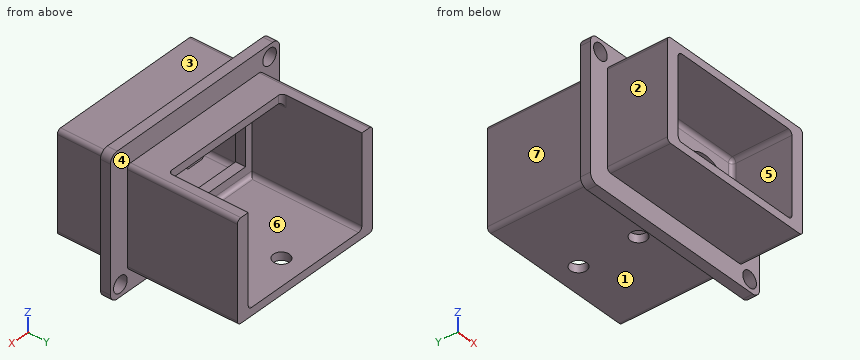
from build123d import *

# Parameters (mm, degrees)
SKETCH1_W                = 63.5
SKETCH1_H                = 44.45
BOSS_EXTRUDE1_DEPTH      = 3.175
FILLET3_R                = 2.54
BOSS_EXTRUDE3_DEPTH      = 19.05
BOSS_EXTRUDE3_DEPTH_BACK = 38.1
SKETCH3_W                = 50.8
SKETCH3_H                = 31.75
SKETCH3_W_2              = 42.672
SKETCH3_H_2              = 26.67
FILLET4_R                = 1.27
SKETCH4_W                = 42.672
SKETCH4_H                = 2.54
CUT_EXTRUDE1_DEPTH       = 25.4
FILLET5_R                = 1.27
FILLET6_R                = 1.27
CUT_EXTRUDE2_REACH       = 64.54
SKETCH5_R                = 2.5527
CUT_EXTRUDE3_REACH       = 56.347
SKETCH6_R                = 2.5527
FILLET7_R                = 1.27


with BuildPart() as part:
    # Sketch1 → Boss-Extrude1 (new body)
    with BuildSketch(Plane(origin=(0, 0, 0), x_dir=(1, 0, 0), z_dir=(0, 1, 0))):
        Rectangle(SKETCH1_W, SKETCH1_H)
        with BuildLine():
            Line((-19.05, -4.014611111), (-19.05, 9.525))
            Line((-19.05, 9.525), (19.05, 9.525))
            Line((19.05, 9.525), (19.05, -4.014611111))
            ThreePointArc((19.05, -4.014611111), (10.305774977, -9.455933485), (3.302, -1.905))
            Line((3.302, -1.905), (-3.302, -1.905))
            ThreePointArc((-3.302, -1.905), (-10.305774977, -9.455933485), (-19.05, -4.014611111))
        make_face(mode=Mode.SUBTRACT)
    extrude(amount=BOSS_EXTRUDE1_DEPTH)

    # Fillet3
    fillet3_edges = [part.edges().sort_by_distance(p)[0] for p in [
        (-31.75, 1.5875, 22.225),
        (-31.75, 1.5875, -22.225),
        (31.75, 1.5875, -22.225),
        (31.75, 1.5875, 22.225),
    ]]
    fillet(fillet3_edges, radius=FILLET3_R)

    # Sketch3 → Boss-Extrude3 (add, two sides: drawn at the far end of the back side and taken through both)
    with BuildSketch(Plane.XZ.offset(-BOSS_EXTRUDE3_DEPTH_BACK)):
        Rectangle(SKETCH3_W, SKETCH3_H)
        Rectangle(SKETCH3_W_2, SKETCH3_H_2, mode=Mode.SUBTRACT)
    extrude(amount=BOSS_EXTRUDE3_DEPTH + BOSS_EXTRUDE3_DEPTH_BACK)

    # Fillet4
    fillet4_edges = [part.edges().sort_by_distance(p)[0] for p in [
        (0, 0, -13.335),
        (21.336, 0, 0),
        (0, 0, 13.335),
        (-21.336, 0, 0),
        (-25.4, -9.525, -15.875),
        (-25.4, -9.525, 15.875),
        (25.4, -9.525, 15.875),
        (25.4, -9.525, -15.875),
        (-21.336, -9.525, 13.335),
        (21.336, -9.525, 13.335),
        (21.336, -9.525, -13.335),
        (-21.336, -9.525, -13.335),
    ]]
    fillet(fillet4_edges, radius=FILLET4_R)

    # Sketch4 → Cut-Extrude1 (cut)
    with BuildSketch(Plane(origin=(0, 38.1, 0), x_dir=(1, 0, 0), z_dir=(0, 1, 0))):
        with Locations((0, -14.605)):
            Rectangle(SKETCH4_W, SKETCH4_H)
    extrude(amount=-CUT_EXTRUDE1_DEPTH, mode=Mode.SUBTRACT)

    # Fillet5
    fillet5_edges = [part.edges().sort_by_distance(p)[0] for p in [
        (21.336, 12.7, 14.605),
        (-21.336, 12.7, 14.605),
        (-3.302, 1.5875, 1.905),
        (3.302, 1.5875, 1.905),
        (0, 3.175, -13.335),
        (21.336, 20.6375, -13.335),
        (-21.336, 20.6375, -13.335),
    ]]
    fillet(fillet5_edges, radius=FILLET5_R)

    # Fillet6
    fillet6_edges = [part.edges().sort_by_distance(p)[0] for p in [
        (0, 3.175, 13.335),
        (-21.336, 8.5725, 13.335),
        (21.336, 8.5725, 13.335),
    ]]
    fillet(fillet6_edges, radius=FILLET6_R)

    # Sketch5 → Cut-Extrude2 (cut, up to next)
    with BuildSketch(Plane(origin=(0, 0, -15.875), x_dir=(-1, 0, 0), z_dir=(0, 0, -1)), mode=Mode.PRIVATE) as cut_extrude2_sk1:
        with Locations((0, 11.557)):
            Circle(SKETCH5_R)
    cut_extrude2_tool1 = extrude(cut_extrude2_sk1.sketch, amount=-CUT_EXTRUDE2_REACH, mode=Mode.PRIVATE) & part.part
    # Sketch5 → Cut-Extrude2 (cut, up to next)
    with BuildSketch(Plane(origin=(0, 0, -15.875), x_dir=(-1, 0, 0), z_dir=(0, 0, -1)), mode=Mode.PRIVATE) as cut_extrude2_sk2:
        with Locations((0, 30.607)):
            Circle(SKETCH5_R)
    cut_extrude2_tool2 = extrude(cut_extrude2_sk2.sketch, amount=-CUT_EXTRUDE2_REACH, mode=Mode.PRIVATE) & part.part
    add(cut_extrude2_tool1.solids().sort_by_distance((0, 11.557, -15.875))[0], mode=Mode.SUBTRACT)
    add(cut_extrude2_tool2.solids().sort_by_distance((0, 30.607, -15.875))[0], mode=Mode.SUBTRACT)

    # Sketch6 → Cut-Extrude3 (cut, up to next)
    with BuildSketch(Plane.XZ, mode=Mode.PRIVATE) as cut_extrude3_sk1:
        with Locations(Location((28.017038418, -18.492038418, 0), (0, 0, 270))):
            Circle(SKETCH6_R)
    cut_extrude3_tool1 = extrude(cut_extrude3_sk1.sketch, amount=-CUT_EXTRUDE3_REACH, mode=Mode.PRIVATE) & part.part
    # Sketch6 → Cut-Extrude3 (cut, up to next)
    with BuildSketch(Plane.XZ, mode=Mode.PRIVATE) as cut_extrude3_sk2:
        with Locations(Location((-28.017038418, 18.492038418, 0), (0, 0, 270))):
            Circle(SKETCH6_R)
    cut_extrude3_tool2 = extrude(cut_extrude3_sk2.sketch, amount=-CUT_EXTRUDE3_REACH, mode=Mode.PRIVATE) & part.part
    add(cut_extrude3_tool1.solids().sort_by_distance((28.017038, 0, -18.492038))[0], mode=Mode.SUBTRACT)
    add(cut_extrude3_tool2.solids().sort_by_distance((-28.017038, 0, 18.492038))[0], mode=Mode.SUBTRACT)

    # Fillet7
    fillet7_edges = [part.edges().sort_by_distance(p)[0] for p in [
        (-25.4, 20.6375, -15.875),
        (-25.4, 20.6375, 15.875),
        (25.4, 20.6375, 15.875),
        (25.4, 20.6375, -15.875),
    ]]
    fillet(fillet7_edges, radius=FILLET7_R)


solid = part.part
Build history of the part. All positions in model axes, mm. Face numbers are marked on the shaded views. A direction names the side the tool comes from. Give positions to 0.01 mm unless a question says otherwise; leave off trailing zeros. Write each loop counter-clockwise with the first axis right and the second up, starting at its lowest first coordinate (ties: lowest second). Pieces come first, ordered by that corner, then holes. Notation, with made-up numbers: (-35.75, 17.5) - (10.25, 17.5) arc R21 cw to (10.25, 26.5) - close; hole circle Ø10 at (59, 87). An arc over 180 degrees is marked (long way). Use one line per item in the form item = value. Start each with the question number.
1. Band-saw the part on C-C on y = 26. Write the cut outline in (x, z) (3 decimals), plus the area to 3 significant figures.
2. Probe line 1 (Y direction, x = 0, z = -14); line 2 (X direction, y = 21, z = -7.5); line 3 (X direction, y = 2, z = 6). List the from-to ranges inside material, lowest first. Write a range as [from, to].
3. Two-plate mould, pull along X, no slides. Class the marked faces 4, 5, 6 and 7: released by +X, released by -X, zero draft, split by the parting line, or undercut.
4. 3-axis set-ups, long thin cutter, end or side, ignore diameter. For the marked faces 1, 2 and 3: which of +Z, -Z, +X, -X, +Y, -Y reach the whole face in a straight line?
5. Band-saw the part on D-D on x = 0. Count the separate pieces of the cut face and the enclosed holes in it, plus the area to 3 significant figures.
6. Band-saw the part on B-B on x = 13. Write the cut outline in (y, z) (3 decimals), plus the area to 3 significant figures.
7. Band-saw the part on A-A on y = -14.5. Write the cut outline in (x, z) (3 decimals), plus the area to 3 significant figures.
8. Drop flat-ended pins along their axis: pin 1 Ø9 at (y, z) = (-8, 1.5) entering from -X; pin 2 Ø8 at (x, z) = (-12, 5) entering from +Y; pin 3 Ø8 at (x, y) = (21, -9) entering from +Z (3 decimals); pin 4 Ø5 at (x, z) = (3, 17.5) entering from +Y. Give the stop position or say it passes through.
Conclusion:
q1.outline = (-25.4, -14.605) arc R1.27 ccw to (-24.13, -15.875) - (24.13, -15.875) arc R1.27 ccw to (25.4, -14.605) - (25.4, 14.605) arc R1.27 ccw to (24.13, 15.875) - (21.336, 15.875) - (21.336, -12.065) arc R1.27 cw to (20.066, -13.335) - (-20.066, -13.335) arc R1.27 cw to (-21.336, -12.065) - (-21.336, 15.875) - (-24.13, 15.875) arc R1.27 ccw to (-25.4, 14.605) - close
q1.area = 366 mm²
q2.line_1 = [-19.05, 9], [14.11, 28.05], [33.16, 38.1]
q2.line_2 = [-25.4, -21.34], [21.34, 25.4]
q2.line_3 = [-31.75, -18.06], [-4.7, 4.7], [18.06, 31.75]
q3.face_4 = zero draft
q3.face_5 = undercut
q3.face_6 = undercut
q3.face_7 = released by -X
q4.face_1 = -Z, +X, -X, +Y
q4.face_2 = +Z, -Z, -X, -Y
q4.face_3 = +Z, +X, -X, -Y
q5.separate_pieces = 4
q5.enclosed_holes = 0
q5.area = 290 mm²
q6.outline = (-19.05, -15.875) - (0, -15.875) - (0, -22.225) - (3.175, -22.225) - (3.175, -15.875) - (38.1, -15.875) - (38.1, -13.335) - (4.445, -13.335) arc R1.27 cw to (3.175, -12.065) - (3.175, -9.525) - (0, -9.525) - (0, -12.065) arc R1.27 cw to (-1.27, -13.335) - (-19.05, -13.335) - close; (-19.05, 13.335) - (-1.27, 13.335) arc R1.27 cw to (0, 12.065) - (0, 9.364) - (3.175, 9.364) - (3.175, 12.065) arc R1.27 cw to (4.445, 13.335) - (12.7, 13.335) - (12.7, 15.875) - (3.175, 15.875) - (3.175, 22.225) - (0, 22.225) - (0, 15.875) - (-19.05, 15.875) - close
q6.area = 292 mm²
q7.outline = (-25.4, -14.605) arc R1.27 ccw to (-24.13, -15.875) - (24.13, -15.875) arc R1.27 ccw to (25.4, -14.605) - (25.4, 14.605) arc R1.27 ccw to (24.13, 15.875) - (-24.13, 15.875) arc R1.27 ccw to (-25.4, 14.605) - close; hole (-21.336, -12.065) arc R1.27 ccw to (-20.066, -13.335) - (20.066, -13.335) arc R1.27 ccw to (21.336, -12.065) - (21.336, 12.065) arc R1.27 ccw to (20.066, 13.335) - (-20.066, 13.335) arc R1.27 ccw to (-21.336, 12.065) - close
q7.area = 475 mm²
q8.pin_1 = -25.4
q8.pin_2 = through
q8.pin_3 = 15.875
q8.pin_4 = 12.7
